Source: CAD feature listing. Evaluate the final solid. Frame: model axes, mm. Give positions to 0.01 mm unless a question says otherwise; leave off trailing zeros. Order: outer loops, then holes, each group sorted by start corner. A loop starts at its lowest first (then second) coordinate and runs counter-clockwise, first axis right, second up.
from build123d import *

# Parameters (mm, degrees)
SKETCH1_W                   = 76.2
SKETCH1_H                   = 298.45
BOSS_EXTRUDE1_DEPTH         = 6.35
F_1_4_20_TAPPED_HOLE1_D     = 5.1054
F_1_4_20_TAPPED_HOLE1_DEPTH = 6.35
CUT_EXTRUDE1_DEPTH          = 7.35
F_0_257_DIAMETER_HOLE1_D    = 6.5278


with BuildPart() as part:
    # Sketch1 → Boss-Extrude1 (new body)
    with BuildSketch(Plane.XY):
        Rectangle(SKETCH1_W, SKETCH1_H)
    extrude(amount=BOSS_EXTRUDE1_DEPTH)

    # 1/4-20 Tapped Hole1
    with Locations(Plane(origin=(0, 0, 0), x_dir=(-1, 0, 0), z_dir=(0, 0, -1))):
        with Locations((-25.4, 130.175), (25.4, 130.175), (25.4, -47.625), (25.4, -123.825), (-25.4, -123.825), (-25.4, -47.625)):
            Hole(F_1_4_20_TAPPED_HOLE1_D / 2, depth=F_1_4_20_TAPPED_HOLE1_DEPTH)

    # Sketch6 → Cut-Extrude1 (cut, through all)
    with BuildSketch(Plane(origin=(0, 0, 0), x_dir=(-1, 0, 0), z_dir=(0, 0, -1))):
        with BuildLine():
            Line((-38.1, 98.425), (-38.1, 0))
            ThreePointArc((-38.1, 0), (-14.729538295, 49.2125), (-38.1, 98.425))
        make_face()
        with BuildLine():
            Line((38.1, 98.425), (38.1, 0))
            ThreePointArc((38.1, 0), (14.729538295, 49.2125), (38.1, 98.425))
        make_face()
    extrude(amount=-CUT_EXTRUDE1_DEPTH, mode=Mode.SUBTRACT)

    # F (0.257) Diameter Hole1 (through all)
    with Locations(Plane(origin=(0, 0, 0), x_dir=(-1, 0, 0), z_dir=(0, 0, -1))):
        with Locations((-25.4, -47.625), (25.4, -47.625), (25.4, -123.825), (-25.4, -123.825)):
            Hole(F_0_257_DIAMETER_HOLE1_D / 2)


solid = part.part
1) Section query A-A on x = 25.4. Output: boundary loops of the cut face in (y, z) (3 decimals), and give its area (3 significant figures).
Checks:
outline: (-149.225, 0) - (-127.089, 0) - (-127.089, 6.35) - (-149.225, 6.35) - close; (-120.561, 0) - (-50.889, 0) - (-50.889, 6.35) - (-120.561, 6.35) - close; (-44.361, 0) - (13.981, 0) - (13.981, 6.35) - (-44.361, 6.35) - close; (84.444, 0) - (127.622, 0) - (127.622, 6.35) - (84.444, 6.35) - close; (132.728, 0) - (149.225, 0) - (149.225, 6.35) - (132.728, 6.35) - close
area: 1,330 mm2
2) Pull-direction query (Y, two-part tool) for faces 1 (the face through (-14.734, 48.424, 3.131)), 2 (the face through (-1, -149.225, 3)), 3 (the face through (24.847, 127.683, 3.219)), 4 (the face through (-38.1, 123, 3)); classes: +Y half, -Y half, draft (parallel to the pull), parting line (faces both ways), or undercut.
Checks:
face 1: undercut
face 2: -Y half
face 3: undercut
face 4: draft
3) Ray query, L1, parallel to Y at x = -24, z = 5.5 (3 decimals); L2, parallel to Y at x = 25.4, z = 3 (3 decimals); L3, parallel to Y at x = -31.5, z = 0.5 (3 decimals). Return the intervals inside material, ascending.
Checks:
L1: y = -149.225 to -126.773, -120.877 to -50.573, -44.677 to 16.176, 82.249 to 128.04, 132.31 to 149.225
L2: y = -149.225 to -127.089, -120.561 to -50.889, -44.361 to 13.981, 84.444 to 127.622, 132.728 to 149.225
L3: y = -149.225 to 6.217, 92.208 to 149.225
4) First-contact query: pin 1 Ø1.5 at (y, z) = (1, 2.5) entering from +X. Flat tip, straight axial feed; report the tip coordinate or a pass-through.
Checks:
pin 1: stops at x = 37.8
5) Section query B-B on z = 4. Output: boundary loops of the cut face in (x, y) (1 decimal).
Checks:
outline: (-38.1, -149.2) - (38.1, -149.2) - (38.1, 0) arc R63.5 cw to (38.1, 98.4) - (38.1, 149.2) - (-38.1, 149.2) - (-38.1, 98.4) arc R63.5 cw to (-38.1, 0) - close; hole circle Ø6.5 at (-25.4, -123.8); hole circle Ø6.5 at (-25.4, -47.6); hole circle Ø5.1 at (-25.4, 130.2); hole circle Ø6.5 at (25.4, -123.8); hole circle Ø6.5 at (25.4, -47.6); hole circle Ø5.1 at (25.4, 130.2)
